Autodesk Inventor part; units mm, degrees
ref_plane "YZ Plane" through (0, 0, 0) normal (1, 0, 0) x (0, 1, 0)
ref_plane "XZ Plane" through (0, 0, 0) normal (0, 1, 0) x (-1, 0, 0)
ref_plane "XY Plane" through (0, 0, 0) normal (0, 0, 1) x (1, 0, 0)
sketch "Эскиз1" plane through (0, 0, 0) normal (0, 0, 1) x (1, 0, 0)
  line L0 (-0.992, 110.468) -> (-0.992, 49.381)
  line L1 (-0.992, 49.381) -> (-0.8881, 48.5921)
  line L2 (-0.8881, 48.5921) -> (-0.5836, 47.857)
  line L3 (-0.5836, 47.857) -> (-0.0993, 47.2257)
  line L4 (-0.0993, 47.2257) -> (0.532, 46.7414)
  line L5 (0.532, 46.7414) -> (1.2671, 46.4369)
  line L6 (1.2671, 46.4369) -> (2.056, 46.333)
  line L7 (2.056, 46.333) -> (23.9, 46.333)
  line L8 (23.9, 46.333) -> (24.4259, 46.4022)
  line L9 (24.4259, 46.4022) -> (24.916, 46.6052)
  line L10 (24.916, 46.6052) -> (25.3368, 46.9282)
  line L11 (25.3368, 46.9282) -> (25.6598, 47.349)
  line L12 (25.6598, 47.349) -> (25.8628, 47.8391)
  line L13 (25.8628, 47.8391) -> (25.932, 48.365)
  line L14 (25.932, 48.365) -> (25.932, 109.579)
  line L15 (25.932, 109.579) -> (25.8195, 110.4336)
  line L16 (25.8195, 110.4336) -> (25.4896, 111.23)
  line L17 (25.4896, 111.23) -> (24.9649, 111.9139)
  line L18 (24.9649, 111.9139) -> (24.281, 112.4386)
  line L19 (24.281, 112.4386) -> (23.4846, 112.7685)
  line L20 (23.4846, 112.7685) -> (22.63, 112.881)
  line L21 (22.63, 112.881) -> (1.421, 112.881)
  line L22 (1.421, 112.881) -> (0.7965, 112.7988)
  line L23 (0.7965, 112.7988) -> (0.2145, 112.5577)
  line L24 (0.2145, 112.5577) -> (-0.2852, 112.1742)
  line L25 (-0.2852, 112.1742) -> (-0.6687, 111.6745)
  line L26 (-0.6687, 111.6745) -> (-0.9098, 111.0925)
  line L27 (-0.9098, 111.0925) -> (-0.992, 110.468)
  circle A0 centre (-26.67, 99.06) radius 0.5
  circle A1 centre (-26.67, 96.52) radius 0.5
  circle A2 centre (-26.67, 93.98) radius 0.5
  circle A3 centre (-26.67, 91.44) radius 0.5
  circle A4 centre (-26.67, 104.14) radius 0.5
  circle A5 centre (-26.67, 88.9) radius 0.5
  circle A6 centre (-26.67, 86.36) radius 0.5
  circle A7 centre (-26.67, 106.68) radius 0.5
  circle A8 centre (-3.81, 63.5) radius 0.5
  circle A9 centre (-26.67, 83.82) radius 0.5
  circle A10 centre (-26.67, 81.28) radius 0.5
  circle A11 centre (-26.67, 78.74) radius 0.5
  circle A12 centre (-26.67, 76.2) radius 0.5
  circle A13 centre (-26.67, 73.66) radius 0.5
  circle A14 centre (-26.67, 71.12) radius 0.5
  circle A15 centre (-26.67, 68.58) radius 0.5
  circle A16 centre (-26.67, 66.04) radius 0.5
  circle A17 centre (-26.67, 63.5) radius 0.5
  circle A18 centre (-26.67, 60.96) radius 0.5
  circle A19 centre (-3.81, 88.9) radius 0.5
  circle A20 centre (-3.81, 86.36) radius 0.5
  circle A21 centre (-3.81, 83.82) radius 0.5
  circle A22 centre (-3.81, 81.28) radius 0.5
  circle A23 centre (-3.81, 78.74) radius 0.5
  circle A24 centre (-3.81, 76.2) radius 0.5
  circle A25 centre (-3.81, 73.66) radius 0.5
  circle A26 centre (-3.81, 71.12) radius 0.5
  circle A27 centre (-3.81, 68.58) radius 0.5
  circle A28 centre (-3.81, 66.04) radius 0.5
  circle A29 centre (-3.81, 60.96) radius 0.5
  circle A30 centre (-3.81, 96.52) radius 0.5
  circle A31 centre (-26.67, 101.6) radius 0.5
  circle A32 centre (-3.81, 104.14) radius 0.5
  circle A33 centre (-3.81, 101.6) radius 0.5
  circle A34 centre (-3.81, 91.44) radius 0.5
  circle A35 centre (-26.67, 109.22) radius 0.5
  circle A36 centre (-3.81, 99.06) radius 0.5
  circle A37 centre (-3.81, 109.22) radius 0.5
  circle A38 centre (-3.81, 106.68) radius 0.5
  circle A39 centre (-3.81, 93.98) radius 0.5
  circle A40 centre (1.02, 92.33) radius 0.5
  circle A41 centre (1.02, 89.79) radius 0.5
  circle A42 centre (1.02, 87.25) radius 0.5
  circle A43 centre (1.02, 84.71) radius 0.5
  circle A44 centre (1.02, 97.41) radius 0.5
  circle A45 centre (1.02, 82.17) radius 0.5
  circle A46 centre (1.02, 79.63) radius 0.5
  circle A47 centre (1.02, 99.95) radius 0.5
  circle A48 centre (23.88, 56.77) radius 0.5
  circle A49 centre (1.02, 77.09) radius 0.5
  circle A50 centre (1.02, 74.55) radius 0.5
  circle A51 centre (1.02, 72.01) radius 0.5
  circle A52 centre (1.02, 69.47) radius 0.5
  circle A53 centre (1.02, 66.93) radius 0.5
  circle A54 centre (1.02, 64.39) radius 0.5
  circle A55 centre (1.02, 61.85) radius 0.5
  circle A56 centre (1.02, 59.31) radius 0.5
  circle A57 centre (1.02, 56.77) radius 0.5
  circle A58 centre (1.02, 54.23) radius 0.5
  circle A59 centre (23.88, 82.17) radius 0.5
  circle A60 centre (23.88, 79.63) radius 0.5
  circle A61 centre (23.88, 77.09) radius 0.5
  circle A62 centre (23.88, 74.55) radius 0.5
  circle A63 centre (23.88, 72.01) radius 0.5
  circle A64 centre (23.88, 69.47) radius 0.5
  circle A65 centre (23.88, 66.93) radius 0.5
  circle A66 centre (23.88, 64.39) radius 0.5
  circle A67 centre (23.88, 61.85) radius 0.5
  circle A68 centre (23.88, 59.31) radius 0.5
  circle A69 centre (23.88, 54.23) radius 0.5
  circle A70 centre (23.88, 89.79) radius 0.5
  circle A71 centre (1.02, 94.87) radius 0.5
  circle A72 centre (23.88, 97.41) radius 0.5
  circle A73 centre (23.88, 94.87) radius 0.5
  circle A74 centre (23.88, 84.71) radius 0.5
  circle A75 centre (1.02, 102.49) radius 0.5
  circle A76 centre (23.88, 92.33) radius 0.5
  circle A77 centre (23.88, 102.49) radius 0.5
  circle A78 centre (23.88, 99.95) radius 0.5
  circle A79 centre (23.88, 87.25) radius 0.5
extrude "untitled.brdКонтур" add sketch "Эскиз1" along normal blind 1.6
sketch "Эскиз2" plane through (-0.992, 49.381, 0) normal (-1, 0, 0) x (0, 0, 1)
  line L0 (-26.1671, -21.9018) -> (16.6735, -21.9018)
  line L1 (16.6735, -21.9018) -> (16.6735, 72.0181)
  line L2 (16.6735, 72.0181) -> (-26.1671, 72.0181)
  line L3 (-26.1671, 72.0181) -> (-26.1671, -21.9018)
  point P0 (0, -49.381)
extrude "Выдавливание2" cut sketch "Эскиз2" along normal blind 30.75
properties part number "untitled.brdКонтур"
CAD build for the part. Positions are in the model's coordinates, mm. Coordinates: 2 decimals unless noted, no trailing zeros.
Item 1: Band-saw the part on A-A on z = 0.35. Give the number of separate pieces and of enclosed holes in the cut face, plus the area to 3 significant figures.
Check sheet entries:
separate pieces: 1
enclosed holes: 40
area: 1,750 mm2
Item 2: Pin check, flat tip, straight feed: pin 1 Ø2 at (x, y) = (8, 77.5) entering from -Z. Stop position of the tip, or through.
Check sheet entries:
pin 1: stops at z = 0
Item 3: Drill centre lines: L1, parallel to X at y = 97.41, z = 1.1; L2, parallel to X at y = 94.5, z = 0.55. Where is each one in solid material? Low to high.
Check sheet entries:
L1: x = -0.99 to 0.52, 1.52 to 23.38, 24.38 to 25.93
L2: x = -0.99 to 0.68, 1.36 to 23.54, 24.22 to 25.93
